```python
from build123d import *

# Parameters (mm, degrees)
BOSS_EXTRUDE1_DEPTH        = 50.8
M3X0_5_TAPPED_HOLE1_D      = 2.5
M3X0_5_TAPPED_HOLE1_DEPTH  = 7.493
M3X0_5_TAPPED_HOLE1_TIP    = 0.751075774
SKETCH8_W                  = 12.7
SKETCH8_H                  = 9.525
SKETCH8_H_2                = 6.35
CUT_EXTRUDE1_DEPTH         = 7.35
F_10_CLEARANCE_HOLE1_D     = 5.1054
F_10_CLEARANCE_HOLE1_DEPTH = 6.35


with BuildPart() as part:
    # Sketch1 → Boss-Extrude1 (new body)
    with BuildSketch(Plane(origin=(0, 0, 0), x_dir=(1, 0, 0), z_dir=(0, 1, 0))):
        Polygon((0, 0), (0, -19.05), (6.35, -19.05), (6.35, -6.35), (15.875, -6.35), (15.875, 0), align=None)
    extrude(amount=BOSS_EXTRUDE1_DEPTH)

    # M3x0.5 Tapped Hole1
    with Locations(Plane.XY.offset(19.05)):
        with Locations((3.175, 38.1), (3.175, 12.7), (3.175, 19.05), (3.175, 31.75)):
            Hole(M3X0_5_TAPPED_HOLE1_D / 2, depth=M3X0_5_TAPPED_HOLE1_DEPTH)
            with Locations((0, 0, -(M3X0_5_TAPPED_HOLE1_DEPTH + M3X0_5_TAPPED_HOLE1_TIP / 2))):  # 118° drill point
                Cone(0, M3X0_5_TAPPED_HOLE1_D / 2, M3X0_5_TAPPED_HOLE1_TIP, mode=Mode.SUBTRACT)

    # Sketch8 → Cut-Extrude1 (cut, through all)
    with BuildSketch(Plane(origin=(6.35, 0, 0), x_dir=(0, 0, -1), z_dir=(1, 0, 0))):
        with Locations((-12.7, 4.7625)):
            Rectangle(SKETCH8_W, SKETCH8_H)
        with Locations((-12.7, 46.0375)):
            Rectangle(SKETCH8_W, SKETCH8_H)
        with Locations((-12.7, 25.4)):
            Rectangle(SKETCH8_W, SKETCH8_H_2)
    extrude(amount=-CUT_EXTRUDE1_DEPTH, mode=Mode.SUBTRACT)

    # #10 Clearance Hole1
    with Locations(Plane.XY.offset(6.35)):
        with Locations((9.525, 6.35), (9.525, 25.4), (9.525, 44.45)):
            Hole(F_10_CLEARANCE_HOLE1_D / 2, depth=F_10_CLEARANCE_HOLE1_DEPTH)


solid = part.part
```
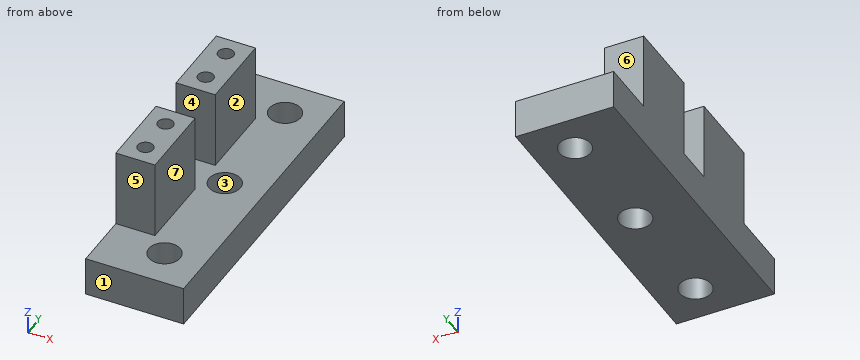
Read the model definition and answer for the solid it produces. Units are mm, in the model's axes. Face numbers are marked on the shaded views. A direction names the side the tool comes from. Round coordinates to 2 decimals unless told otherwise and drop trailing zeros. Write each loop counter-clockwise with the first axis right and the second up, starting at its lowest first coordinate (ties: lowest second). Pieces come first, ordered by that corner, then holes. Notation, with made-up numbers: (84, -23.5) - (96, -23.5) arc R22 cw to (96, -9.5) - close; hole circle Ø3 at (61.5, 63.5). An arc over 180 degrees is marked (long way). One line per item, written item: value.
Q1. Each of these flat-tipped pins is pushed along its axis until it touches: P1, Ø6.5, axis at x = 9.525, y = 44.45, coming from the +Z side; P2, Ø8, axis at x = 9.5, y = 27, coming from the +Z side; P3, Ø4, axis at y = 36.5, z = 12.5, coming from the +X side; P4, Ø3, axis at x = 3.5, z = 15.5, coming from the -Y side (3 decimals). Where does it stop, or does it pass through?
The answers:
P1: stops at z = 6.35
P2: stops at z = 19.05
P3: stops at x = 6.35
P4: stops at y = 9.525
Q2. Find section D-D (z = 4.75). Determine the outline of the cut face in (x, y) (3 decimals).
The answers:
outline: (0, 0) - (15.875, 0) - (15.875, 50.8) - (0, 50.8) - close; hole circle Ø5.105 at (9.525, 6.35); hole circle Ø5.105 at (9.525, 25.4); hole circle Ø5.105 at (9.525, 44.45)
Q3. For a pull along X with two mould halves and no side action, classify the marked faces 1, 2 and 3 as pulls with the +X half, pulls with the -X half, needs draft (parallel to the pull), parting line crosses it, or undercut.
The answers:
face 1: needs draft
face 2: pulls with the +X half
face 3: undercut
Q4. Straight lines are drawn through the part: line 1 (Y direction, x = 5.25, z = 10.25) (3 decimals); line 2 (Y direction, x = 7.5, z = 5); line 3 (X direction, y = 38.1, z = 13.75) (3 decimals). For each, find the intervals that lie inside material, in ascending order. Write a range as from..to.
The answers:
line 1: y = 9.525..22.225, 28.575..41.275
line 2: y = 0..4.8, 7.9..23.85, 26.95..42.9, 46..50.8
line 3: x = 0..1.925, 4.425..6.35
Q5. Find section C-C (x = 5.75). Determine the outline of the cut face in (y, z) (3 decimals).
The answers:
outline: (0, 0) - (50.8, 0) - (50.8, 6.35) - (41.275, 6.35) - (41.275, 19.05) - (28.575, 19.05) - (28.575, 6.35) - (22.225, 6.35) - (22.225, 19.05) - (9.525, 19.05) - (9.525, 6.35) - (0, 6.35) - close
Q6. Find section B-B (y = 44.45). Determine the outline of the cut face in (x, z) (3 decimals).
The answers:
outline: (0, 0) - (6.972, 0) - (6.972, 6.35) - (0, 6.35) - close; (12.078, 0) - (15.875, 0) - (15.875, 6.35) - (12.078, 6.35) - close
Q7. Find section A-A (z = 15). Determine the outline of the cut face in (x, y) (3 decimals).
The answers:
outline: (0, 9.525) - (6.35, 9.525) - (6.35, 22.225) - (0, 22.225) - close; (0, 28.575) - (6.35, 28.575) - (6.35, 41.275) - (0, 41.275) - close; hole circle Ø2.5 at (3.175, 12.7); hole circle Ø2.5 at (3.175, 19.05); hole circle Ø2.5 at (3.175, 31.75); hole circle Ø2.5 at (3.175, 38.1)
Q8. Which of the six approach directions +Z, -Z, +X, -X, +Y, -Y give full straight-line access (tool end or side, diameter ignored) to the marked faces 4, 5, 6 and 7?
The answers:
face 4: +Z, +X, -X
face 5: +Z, +X, -X, -Y
face 6: +Z, +X, -X, +Y
face 7: +Z, +X, +Y, -Y
